Verification items for the finished model (mm, model axes). A direction names the side the tool comes from. Give positions to 0.01 mm unless a question says otherwise; leave off trailing zeros. Loops run counter-clockwise (first coordinate to the right, second up) from the corner with the lowest first, then second, coordinate; pieces in that order, holes last. Notation, with made-up numbers: (-33.5, 10) - (20.5, 10) arc R26 ccw to (20.5, 33) - close; hole circle Ø9 at (-1, 37.5). An arc over 180 degrees is marked (long way). One line per item, written item: value. Start each with the question number.
1. Mould release check, pull along X, two halves, no side actions. Record for faces 1 (the flat face through (50.8, 10, -15)), 2 (the cylindrical face through (28.43, 18.84, 0.95)), 3 (the flat face through (0, 10, -15)): pulls with the +X half, pulls with the -X half, needs draft (parallel to the pull), parting line crosses it, or undercut.
2. Sectioned sample at C-C (y = 6). Record the cut outline in (x, z), plus the area to 3 significant figures.
3. Gauge pin test, flat ends, axial feed: pin 1 (5 mm diameter, centred on y = -9.5, z = 95.5, fed in from -X); pin 2 (3 mm diameter, centred on x = 17.5, z = 11.5, fed in from -Y); pin 3 (8 mm diameter, centred on y = 6, z = 45, fed in from +X). Record the tip position at first contact, or that the pin passes through.
4. Access from +Z, -Z, +X, -X, +Y, -Y to the whole of each face (thin tool, end or side, straight path). Record for faces 4 (the flat face through (25, -12.7, 72)), 5 (the flat face through (26, 12.7, 72)), 6 (the flat face through (25, 0, 127)).
5. Scan lines: L1, parallel to X at y = 17.75, z = 0 (3 decimals); L2, parallel to Y at x = 40.5, z = 0 (3 decimals); L3, parallel to Z at x = 9, y = -2.5. Record each from-to range of solid material in increasing order. Write a range as [from, to].
6. Sectioned sample at A-A (x = 20). Record the cut outline in (y, z) (3 decimals).
7. Sectioned sample at B-B (z = 99.5). Record the cut outline in (x, y), plus the area to 3 significant figures.
from build123d import *
from build123d import SkipClean  # not in build123d's __all__

# Parameters (mm, degrees)
F0_R     = 22.225
F0_R_2   = 15.875
F1_DEPTH = 50.8
F2_R     = 3.175
F3_DEPTH = 37.592
F5_DEPTH = 127
F6_R     = 15.875
F7_DEPTH = 70.104


with BuildPart() as f1:
    # F0 (on Right) → F1 (new body)
    with BuildSketch(Plane.YZ):
        Circle(F0_R)
        Circle(F0_R_2, mode=Mode.SUBTRACT)
    extrude(amount=F1_DEPTH)

    # F2 (on Front) → F3 (cut)
    with BuildSketch(Plane.XZ):
        with Locations((25.4, 0)):
            Circle(F2_R)
    extrude(amount=-F3_DEPTH, mode=Mode.SUBTRACT)

    # F4 (on Top) → F5 (join)
    with BuildSketch(Plane.XY):
        with BuildLine():
            ThreePointArc((12.7, 12.7), (3.7197438789, 8.9802561211), (0, 0))
            Line((0, 0), (12.7, 0))
            Line((12.7, 0), (12.7, 12.7))
        make_face()
        with BuildLine():
            Line((12.7, 0), (0, 0))
            ThreePointArc((0, 0), (3.7197438789, -8.9802561211), (12.7, -12.7))
            Line((12.7, -12.7), (12.7, 0))
        make_face()
        with BuildLine():
            Line((12.7, 12.7), (12.7, 0))
            Line((12.7, 0), (25.4, 0))
            ThreePointArc((25.4, 0), (21.6802561211, 8.9802561211), (12.7, 12.7))
        make_face()
        with BuildLine():
            Line((25.4, 0), (12.7, 0))
            Line((12.7, 0), (12.7, -12.7))
            ThreePointArc((12.7, -12.7), (21.6802561211, -8.9802561211), (25.4, 0))
        make_face()
        with BuildLine():
            Line((38.1, 12.7), (12.7, 12.7))
            ThreePointArc((12.7, 12.7), (21.6802561211, 8.9802561211), (25.4, 0))
            ThreePointArc((25.4, 0), (29.1197438789, 8.9802561211), (38.1, 12.7))
        make_face()
        with BuildLine():
            ThreePointArc((25.4, 0), (21.6802561211, -8.9802561211), (12.7, -12.7))
            Line((12.7, -12.7), (38.1, -12.7))
            ThreePointArc((38.1, -12.7), (29.1197438789, -8.9802561211), (25.4, 0))
        make_face()
        with BuildLine():
            ThreePointArc((38.1, 12.7), (29.1197438789, 8.9802561211), (25.4, 0))
            Line((25.4, 0), (38.1, 0))
            Line((38.1, 0), (38.1, 12.7))
        make_face()
        with BuildLine():
            Line((38.1, 0), (25.4, 0))
            ThreePointArc((25.4, 0), (29.1197438789, -8.9802561211), (38.1, -12.7))
            Line((38.1, -12.7), (38.1, 0))
        make_face()
        with BuildLine():
            ThreePointArc((50.8, 0), (47.0802561211, 8.9802561211), (38.1, 12.7))
            Line((38.1, 12.7), (38.1, 0))
            Line((38.1, 0), (38.1, -12.7))
            ThreePointArc((38.1, -12.7), (47.0802561211, -8.9802561211), (50.8, 0))
        make_face()
    with SkipClean():  # cleaning this boolean's faces spoils the solid; the shape is the same uncleaned
        extrude(amount=F5_DEPTH)

    # F6 (on face) → F7 (cut)
    with BuildSketch(Plane.YZ.offset(50.8)):
        Circle(F6_R)
    with SkipClean():  # cleaning this boolean's faces spoils the solid; the shape is the same uncleaned
        extrude(amount=-F7_DEPTH, mode=Mode.SUBTRACT)


solid = f1.part
Results are:
1. face 1: pulls with the +X half
1. face 2: undercut
1. face 3: pulls with the -X half
2. outline: (0, -21.4) - (50.8, -21.4) - (50.8, -14.7) - (0, -14.7) - close; (0, 14.7) - (50.8, 14.7) - (50.8, 21.4) - (49.29, 21.4) - (49.29, 127) - (1.51, 127) - (1.51, 21.4) - (0, 21.4) - close
2. area: 5,730 mm^2
3. pin 1: stops at x = 2.1
3. pin 2: stops at y = -19.85
3. pin 3: stops at x = 50.64
4. face 4: +Z, +X, -X, -Y
4. face 5: +Z, +X, -X, +Y
4. face 6: +Z, +X, -X, +Y, -Y
5. L1: x = [0, 22.225], [28.575, 50.8]
5. L2: y = [-22.225, -15.875], [15.875, 22.225]
5. L3: z = [-22.08, -15.68], [15.68, 127]
6. outline: (-12.7, 18.239) arc R22.225 ccw (long way) to (12.7, 18.239) - (12.7, 127) - (-12.7, 127) - close; hole circle Ø31.75 at (0, 0)
7. outline: (12.7, -12.7) - (38.1, -12.7) arc R12.7 ccw to (38.1, 12.7) - (12.7, 12.7) arc R12.7 ccw to start
7. area: 1,150 mm^2
